Autodesk Inventor part; units mm, degrees
ref_plane "YZ Plane" through (0, 0, 0) normal (1, 0, 0) x (0, 1, 0)
ref_plane "XZ Plane" through (0, 0, 0) normal (0, 1, 0) x (-1, 0, 0)
ref_plane "XY Plane" through (0, 0, 0) normal (0, 0, 1) x (1, 0, 0)
sketch "Sketch1" plane through (0, 0, 0) normal (0, 0, 1) x (1, 0, 0)
  line L0 (-1.3293, 0) -> (17.4625, 0)
  line L1 (17.4625, 0) -> (17.4625, 2.413)
  line L2 (17.4625, 2.413) -> (7.9375, 2.413)
  line L3 (7.9375, 2.413) -> (7.9375, 3.1496)
  line L4 (7.9375, 3.1496) -> (0, 3.1496)
  line L5 (0, 3.1496) -> (0, 4.7625)
  line L6 (0, 4.7625) -> (-4.7752, 4.7625)
  line L7 (-4.7752, 4.7625) -> (-4.7752, 1.8331)
  line L8 (-4.7752, 1.8331) -> (-2.3876, 1.8331)
  line L9 (-2.3876, 1.8331) -> (-1.3293, 0)
  line L10 (-8.9052, 0) -> (20.005, 0)
  line L11 (0, -0.9525) -> (0, 5.715)
  line L12 (0, 2.8829) -> (2.0955, 2.8829)
  line L13 (2.0955, 2.8829) -> (2.3622, 3.1496)
  line L14 (7.9375, 2.413) -> (7.9375, 1.7831)
  line L15 (7.9375, 1.7831) -> (10.0457, 1.7831)
  line L16 (10.0457, 1.7831) -> (10.6756, 2.413)
  line L17 (0, 2.8829) -> (0, 3.1496)
  dimension "d0" = 4.826
  dimension "d1" = 6.2992
  dimension "d2" = 9.525
  dimension "d3" = 3.6662
  dimension "d5" = 9.525
  dimension "d6" = 4.7752
  dimension "d7" = 2.3876
  dimension "d8" = 60
  dimension "d9" = 17.4625
  dimension "d19" = 45
  dimension "d20" = 5.7658
  dimension "d21" = 3.5662
  dimension "d22" = 45
  dimension "d23" = 2.1082
  dimension "d34" = 2.3622
revolve "Body" add sketch "Sketch1" angle 360 about axis through (-1.3293, 0, 0) along (1, 0, 0)
sketch "Sketch2" plane through (-4.7752, 0, 0) normal (-1, 0, 0) x (0, 0, 1)
  circle A0 centre (0, 0) radius 1.8331
  line L0 (0, 1.8331) -> (1.5875, 0.9165)
  line L1 (1.5875, 0.9165) -> (1.5875, -0.9165)
  line L2 (1.5875, -0.9165) -> (0, -1.8331)
  line L3 (0, -1.8331) -> (-1.5875, -0.9165)
  line L4 (-1.5875, -0.9165) -> (-1.5875, 0.9165)
  line L5 (-1.5875, 0.9165) -> (0, 1.8331)
  point P0 (0, 0)
extrude "Slot" add sketch "Sketch2" against normal up to next contours A0 L1 | L0 A0 | A0 L2 | L5 A0 | A0 L3 | L4 A0
fillet "Fillet1" radius 2.3622 1 edges at (-4.7752, -4.7625, 0)
thread "Thread"
chamfer "Chamfer1" distance 0.6299 distance2 0.6299 1 edges at (17.4625, -2.413, 0) measured on face at (17.4625, 0.4138, 0.5798)
chamfer "Chamfer2" distance 0.127 angle 45 1 edges at (7.9375, -3.1496, 0) measured on face at (7.9375, 2.8502, -0.4437)
revolve "Groove1" cut sketch "Sketch1" angle 360 about axis through (-1.3293, 0, 0) along (1, 0, 0) contours L11 L4 L13 L12
revolve "Groove2" cut sketch "Sketch1" angle 360 about axis through (-1.3293, 0, 0) along (1, 0, 0) contours L16 L15 L14 L2
equation "\"d0\" = NND"
equation "\"d1\" = BDM"
equation "\"d2\" = KOD"
equation "\"d3\" = 1.1547 * SW"
equation "\"d5\" = GEL"
equation "\"d6\" = KOH"
equation "\"d7\" = INTI + LOTI"
equation "\"d8\" = 0.5 * ANG"
equation "\"d9\" = NLG"
equation "\"d19\" = FAWI4"
equation "\"d20\" = BDMM"
equation "\"d21\" = GD1"
equation "\"d22\" = FAWI2"
equation "\"d23\" = GAL"
equation "\"d34\" = GAL2"
equation "\"d13\" = RR"
equation "\"d25\" = GEL"
equation "\"d14\" = -0.5 * SPD + 0.5 * NND"
equation "\"d15\" = GUL"
equation "\"d32\" = -0.5 * NND + 0.5 * BDM"
equation "\"NND\" = 4.826"
equation "\"NLG\" = 17.4625"
equation "\"GEL\" = 9.525"
equation "\"KOD\" = 9.525"
equation "\"KOH\" = 4.7752"
equation "\"INTI\" = 2.3876"
equation "\"GAL\" = 2.1082"
equation "\"GUL\" = 0.62992"
equation "\"SPD\" = GD1"
equation "\"BDM\" = 6.2992"
equation "\"ANG\" = 120deg"
equation "\"FAWI2\" = 45deg"
equation "\"FAWI3\" = 45deg"
equation "\"FAWI4\" = 45deg"
equation "\"RR\" = 2.3622"
equation "\"SW\" = 3.175"
equation "\"BDMM\" = 5.7658"
equation "\"GAL2\" = RR"
equation "\"LOTI\" = 0"
equation "\"GD1\" = 3.56616"
equation "\"BOR\" = SW"
equation "\"SLG\" = 6.35"
equation "\"THREADDIA\" = 4.826"
equation "\"E0\" = 1.155 * SW"
equation "\"FAWI1\" = 45deg"
equation "\"TOA\" = 30deg"
equation "\"PHH\" = RR"
equation "\"HHPTC\" = 1.05842"
equation "\"GD0\" = 3.3782"
equation "\"KOH1\" = 3.9878"
equation "\"BDMN\" = 6.35"
properties part number "ANSI B18.3 - 0.250 x 0.25 ANSI B18.3" material "Steel, Mild"
Part model, mm, in its own coordinate system. A direction names the side the tool comes from. Give positions to 0.01 mm unless a question says otherwise; leave off trailing zeros. Write each loop counter-clockwise with the first axis right and the second up, starting at its lowest first coordinate (ties: lowest second). Pieces come first, ordered by that corner, then holes.
1) Which spindle directions (+Z, -Z, +X, -X, +Y, -Y) get a long thin tool onto all of the face, cutting with end or side? Do faces 4 (the face through (-4, 0, -1.588)), 5 (the face through (13.711, -1.915, 1.468)), 6 (the face through (9.01, -0.39, -1.74)). Say none if no direction does.
Resolved:
face 4: -X
face 5: +X
face 6: none
2) Cut at B-B on x = 13. Write the cut outline in (y, z), then the cut area to 3 significant figures.
Resolved:
outline: circle Ø4.83 at (0, 0)
area: 18.3 mm2
3) Cut at C-C on x = 5.75. Write the cut outline in (y, z).
Resolved:
outline: circle Ø6.3 at (0, 0)
4) Pin check, flat tips, straight feed: pin 1 (1.5 mm diameter, centred on x = 15, y = 0, fed in from -Z); pin 2 (1 mm diameter, centred on x = 6.5, y = -4, fed in from -Z); pin 3 (5 mm diameter, centred on x = 12.5, z = -1, fed in from +Y); pin 4 (0.5 mm diameter, centred on x = -3.5, y = 0.5, fed in from -Z). Stop position of each tip, or through.
Resolved:
pin 1: stops at z = -2.41
pin 2: passes through
pin 3: stops at y = 2.41
pin 4: stops at z = -4.59
5) Cut at A-A on x = -3.5. Write the cut outline in (y, z).
Resolved:
outline: circle Ø9 at (0, 0); hole (-1.83, 0) - (-0.92, -1.59) - (0.92, -1.59) - (1.83, 0) - (0.92, 1.59) - (-0.92, 1.59) - close
6) Two-plate mould, pull along X, no slides. Class faces 1 (the face through (7.938, 2, 0)), 2 (the face through (-1.396, -0.025, 0.112)), 3 (the face through (-3.53, 1.37, -0.8)): released by +X, released by -X, zero draft, split by the parting line, or undercut.
Resolved:
face 1: undercut
face 2: released by -X
face 3: zero draft
7) Probe L1, parallel to Z at x = -2.5, y = -1.5; L2, parallel to X at y = 0.25, z = -2.5; L3, parallel to X at y = -0.75, z = -2.25. List the from-to ranges inside material, lowest first.
Resolved:
L1: z = -4.52 to -0.58, 0.58 to 4.52
L2: x = -4.77 to 7.94
L3: x = -4.78 to 7.94, 10.63 to 16.87
